Check sheet for the modelled part. Datum: model origin and axes. Units: mm. A direction names the side the tool comes from. Round coordinates to 2 decimals unless told otherwise and drop trailing zeros. Write each loop counter-clockwise with the first axis right and the second up, starting at its lowest first coordinate (ties: lowest second). Pieces come first, ordered by that corner, then holes. Notation, with made-up numbers: (8.25, 62) -> (43.25, 62) arc R8 ccw to (43.25, 72) -> close; hole circle Ø5 at (83, -5). An arc over 180 degrees is marked (long way). Answer as a JSON object with one key per item and string values. Group by question number.
Autodesk Inventor part; units mm, degrees
ref_plane "YZ Plane" through (0, 0, 0) normal (1, 0, 0) x (0, 1, 0)
ref_plane "XZ Plane" through (0, 0, 0) normal (0, 1, 0) x (-1, 0, 0)
ref_plane "XY Plane" through (0, 0, 0) normal (0, 0, 1) x (1, 0, 0)
sketch "Szkic1" plane through (0, 0, 0) normal (0, 1, 0) x (-1, 0, 0)
  line L0 (3, 7.5) -> (-3, 7.5)
  line L1 (-3, 7.5) -> (-3, -7.5)
  line L2 (-3, -7.5) -> (3, -7.5)
  line L3 (3, -7.5) -> (3, 7.5)
  point P0 (0, 0)
  point P1 (0, -7.5)
  point P2 (3, 0)
  dimension "d0" = 6
  dimension "d1" = 15
extrude "Wyciągnięcie proste1" add sketch "Szkic1" along normal blind 10
sketch "Szkic2" plane through (0, 10, 0) normal (0, 1, 0) x (1, 0, 0)
  circle A0 centre (0, -5) radius 1.95
  circle A1 centre (0, 0) radius 2
  circle A2 centre (0, 5) radius 2.05
  dimension "d4" = 3.9
  dimension "d5" = 4
  dimension "d6" = 4.1
  dimension "d7" = 5
  dimension "d8" = 5
extrude "Wyciągnięcie proste2" cut sketch "Szkic2" against normal blind 9
sketch "Szkic3" plane through (0, 10, 0) normal (0, 1, 0) x (1, 0, 0)
  line L0 (3, -7.5) -> (3, 7.5)
  line L1 (3, -5.2848) -> (2.5823, -5.2848)
  line L2 (2.5823, -5.2848) -> (2.5823, -4.7242)
  line L3 (2.5823, -4.7242) -> (3, -4.7242)
  line L4 (3, -4.7242) -> (3, -5.2848)
  line L5 (3, -0.7206) -> (2.5823, -0.7206)
  line L6 (2.5823, -0.7206) -> (2.5823, -0.2402)
  line L7 (2.5823, -0.2402) -> (3, -0.2402)
  line L8 (3, -0.2402) -> (3, -0.7206)
  line L9 (3, 0.5405) -> (2.5823, 0.5405)
  line L10 (2.5823, 0.5405) -> (2.5823, 1.2211)
  line L11 (2.5823, 1.2211) -> (3, 1.2211)
  line L12 (3, 1.2211) -> (3, 0.5405)
  line L13 (3, 3.7634) -> (2.5823, 3.7634)
  line L14 (2.5823, 3.7634) -> (2.5823, 4.3039)
  line L15 (2.5823, 4.3039) -> (3, 4.3039)
  line L16 (3, 4.3039) -> (3, 3.7634)
  line L17 (3, 4.9244) -> (2.5823, 4.9244)
  line L18 (2.5823, 4.9244) -> (2.5823, 5.4049)
  line L19 (2.5823, 5.4049) -> (3, 5.4049)
  line L20 (3, 5.4049) -> (3, 4.9244)
  line L21 (3, 5.9453) -> (2.5823, 5.9453)
  line L22 (2.5823, 5.9453) -> (2.5823, 6.4858)
  line L23 (2.5823, 6.4858) -> (3, 6.4858)
  line L24 (3, 6.4858) -> (3, 5.9453)
  point P0 (0, 0)
extrude "Wyciągnięcie proste3" cut sketch "Szkic3" against normal blind 5
properties part number "TEST"
(1) Section check D-D on y = 4.5. Record the cut outline in (x, z).
(2) Section check A-A on y = 5.75. State how many separate pieces and enclosed holes the cut face has, then the cut area to 3 significant figures.
(3) Section check C-C on x = 0. Record the cut outline in (y, z), then the cut area to 3 significant figures.
(4) Go/stop test with a flat-tipped pin: pin 1 Ø2 at (x, z) = (0, -4) entering from +Y. Record where the tip stops, or that it passes through.
(5) Scan lines: line 1 along Z through (x, y) = (0, 4.5); line 2 along Z through (x, y) = (-0.5, 6.5); line 3 along X through (y, z) = (1.5, 5). Record each from-to range of solid material in increasing order.
(6) Access from +Z, -Z, +X, -X, +Y, -Y to the whole of each face (thin tool, end or side, straight path). Record for faces 1 (the flat face through (0, 1, 5)), 2 (the flat face through (0, 0, 0)).
(7) Release check for a two-part mould opening along X. For faces 3 (the flat face through (0, 5, -7.5)), 4 (the flat face through (-3, 5, 0)), 5 (the cylindrical face through (0, 6, 2)), 6 (the flat face through (0, 1, 0)) record: pulls with the +X half, pulls with the -X half, needs draft (parallel to the pull), parting line crosses it, or undercut.
(8) Section check B-B on z = 5. Record the cut outline in (x, y).
Data:
{
 "1": {"outline": "(-3, -7.5) -> (3, -7.5) -> (3, 7.5) -> (-3, 7.5) -> close; hole circle Ø4.1 at (0, -5); hole circle Ø4 at (0, 0); hole circle Ø3.9 at (0, 5)"},
 "2": {"separate pieces": "1", "enclosed holes": "3", "area": "50.9 mm²"},
 "3": {"outline": "(0, -7.5) -> (10, -7.5) -> (10, -7.05) -> (1, -7.05) -> (1, -2.95) -> (10, -2.95) -> (10, -2) -> (1, -2) -> (1, 2) -> (10, 2) -> (10, 3.05) -> (1, 3.05) -> (1, 6.95) -> (10, 6.95) -> (10, 7.5) -> (0, 7.5) -> close", "area": "42.0 mm²"},
 "4": {"pin 1": "stops at y = 1"},
 "5": {"line 1": "z = -7.5 to -7.05, -2.95 to -2, 2 to 3.05, 6.95 to 7.5", "line 2": "z = -7.5 to -6.99, -3.01 to -1.94, 1.94 to 3.12, 6.88 to 7.5", "line 3": "x = -3 to -1.95, 1.95 to 3"},
 "6": {"face 1": "+Y", "face 2": "+Z, -Z, +X, -X, -Y"},
 "7": {"face 3": "needs draft", "face 4": "pulls with the -X half", "face 5": "undercut", "face 6": "undercut"},
 "8": {"outline": "(-3, 0) -> (3, 0) -> (3, 5) -> (2.58, 5) -> (2.58, 10) -> (1.95, 10) -> (1.95, 1) -> (-1.95, 1) -> (-1.95, 10) -> (-3, 10) -> close"}
}
